Read the model definition and answer for the solid it produces. Units are mm, in the model's axes. Round coordinates to 2 decimals unless told otherwise and drop trailing zeros. Write each loop counter-clockwise with the first axis right and the second up, starting at its lowest first coordinate (ties: lowest second). Pieces come first, ordered by that corner, then holes.
Autodesk Inventor part; units mm, degrees
ref_plane "YZ Plane" through (0, 0, 0) normal (1, 0, 0) x (0, 1, 0)
ref_plane "XZ Plane" through (0, 0, 0) normal (0, 1, 0) x (-1, 0, 0)
ref_plane "XY Plane" through (0, 0, 0) normal (0, 0, 1) x (1, 0, 0)
sketch "Sketch1" plane through (0, 0, 0) normal (0, 1, 0) x (-1, 0, 0)
  line L0 (8.4467, 22.8129) -> (-5.2472, 22.8129)
  line L1 (-5.2472, 22.8129) -> (-5.2472, -32.1871)
  line L2 (-5.2472, -32.1871) -> (8.4467, -32.1871)
  line L3 (8.4467, -32.1871) -> (8.4467, 22.8129)
  circle A0 centre (5.8231, 19.3129) radius 1.5
  circle A1 centre (5.932, 4.3133) radius 1.5
  circle A2 centre (5.932, -28.6871) radius 1.5
  circle A3 centre (5.932, -13.6871) radius 1.5
  point P0 (0, 0)
  dimension "d0" = 3
  dimension "d1" = 3
  dimension "d2" = 15
  dimension "d3" = 55
  dimension "d4" = 3
  dimension "d5" = 3
  dimension "d6" = 15
  dimension "d7" = 3.5
  dimension "d8" = 3.5
extrude "Extrusion1" add sketch "Sketch1" along normal blind 3
properties part number "soporte"
Q1. Section B-B (x = -6.5) is taken. Determine the outline of the cut face in (y, z) (3 decimals), then the cut area to 3 significant figures.
Verdict:
outline: (0, -32.187) - (3, -32.187) - (3, -30.075) - (0, -30.075) - close; (0, -27.299) - (3, -27.299) - (3, -15.075) - (0, -15.075) - close; (0, -12.299) - (3, -12.299) - (3, 2.925) - (0, 2.925) - close; (0, 5.702) - (3, 5.702) - (3, 17.974) - (0, 17.974) - close; (0, 20.651) - (3, 20.651) - (3, 22.813) - (0, 22.813) - close
area: 132 mm2
Q2. Straight lines are drawn through the part: probe 1 along Z at (x, y) = (-5.75, 2.85); probe 2 along X at (y, z) = (1.9, 19); probe 3 along Z at (x, y) = (-6.25, 2.3). For each, find the intervals that lie inside material, in ascending order.
Verdict:
probe 1: z = -32.19 to -30.18, -27.2 to -15.18, -12.2 to 2.82, 5.8 to 17.81, 20.81 to 22.81
probe 2: x = -8.45 to -7.29, -4.36 to 5.25
probe 3: z = -32.19 to -30.15, -27.22 to -15.15, -12.22 to 2.85, 5.78 to 17.87, 20.75 to 22.81
Q3. Section A-A (y = 1.5) is taken. Determine the outline of the cut face in (x, z), then the cut area to 3 significant figures.
Verdict:
outline: (-8.45, -32.19) - (5.25, -32.19) - (5.25, 22.81) - (-8.45, 22.81) - close; hole circle Ø3 at (-5.93, -28.69); hole circle Ø3 at (-5.93, -13.69); hole circle Ø3 at (-5.93, 4.31); hole circle Ø3 at (-5.82, 19.31)
area: 725 mm2
Q4. Determine the mould class of faces 1 (the flat face through (-8.447, 1, -5)), 2 (the flat face through (-2, 1, -32.187)), 3 (the cylindrical face through (-4.742, 1.479, 5.226)) for opening direction Z: pulls with the +Z half, pulls with the -Z half, needs draft (parallel to the pull), parting line crosses it, or undercut.
Verdict:
face 1: needs draft
face 2: pulls with the -Z half
face 3: undercut
Q5. A flat-ended cylindrical pin translates along its axis: pin 1 Ø4 at (x, z) = (-5.93, 4.31) entering from -Y. Find the tip coordinate at first contact, or state that the pin passes through.
Verdict:
pin 1: stops at y = 0
